from build123d import *

# Parameters (mm, degrees)
SCHIZZO1_W                   = 35
SCHIZZO1_H                   = 25
ESTRUSIONE_ESTRUSIONE1_DEPTH = 50
SCHIZZO2_R                   = 10.25
TAGLIO_ESTRUSIONE1_DEPTH     = 100
SCHIZZO3_R                   = 8.55
TAGLIO_ESTRUSIONE3_DEPTH     = 63.299678972
SMUSSO1_SIZE                 = 0.5


with BuildPart() as part:
    # Schizzo1 → Estrusione-Estrusione1 (new, symmetric)
    with BuildSketch(Plane.XY):
        Rectangle(SCHIZZO1_W, SCHIZZO1_H)
    extrude(amount=ESTRUSIONE_ESTRUSIONE1_DEPTH, both=True)

    # Schizzo2 → Taglio-Estrusione1 (cut)
    with BuildSketch(Plane(origin=(0, 12.5, 0), x_dir=(1, 0, 0), z_dir=(0, 1, 0))):
        with Locations(Location((0, 0, 0), (0, 0, 270))):
            Circle(SCHIZZO2_R)
    extrude(amount=-TAGLIO_ESTRUSIONE1_DEPTH, mode=Mode.SUBTRACT)

    # Schizzo3 → Taglio-Estrusione3 (cut, through all)
    with BuildSketch(Plane(origin=(17.5, 0, 0), x_dir=(0, 0, -1), z_dir=(1, 0, 0))):
        with Locations(Location((37.5, 0, 0), (0, 0, 90))):
            Circle(SCHIZZO3_R)
        with Locations(Location((-37.5, 0, 0), (0, 0, 90))):
            Circle(SCHIZZO3_R)
    extrude(amount=-TAGLIO_ESTRUSIONE3_DEPTH, mode=Mode.SUBTRACT)

    # Smusso1
    smusso1_edges = [part.edges().sort_by_distance(p)[0] for p in [
        (0, -12.5, -10.25),
        (0, 12.5, -10.25),
        (-17.5, -8.55, -37.5),
        (17.5, -8.55, -37.5),
        (-17.5, -8.55, 37.5),
        (17.5, -8.55, 37.5),
    ]]
    chamfer(smusso1_edges, length=SMUSSO1_SIZE)


solid = part.part
Read the model definition and answer for the solid it produces. Units are mm, in the model's axes. Round coordinates to 2 decimals unless told otherwise and drop trailing zeros. Loops run counter-clockwise (first coordinate to the right, second up) from the corner with the lowest first, then second, coordinate; pieces in that order, holes last.
Q1. Section D-D on x = -6 is taken. Give the number of separate pieces and of enclosed holes in the cut face, and give its area (3 significant figures).
Q2. Section A-A on y = 0 is taken. Write down the section's boundary in (x, z).
Q3. Consider probe 1 along X at (y, z) = (7, 0); probe 2 along Z at (x, y) = (5.5, -4); probe 3 along Z at (x, y) = (14, -7.75). Determine where each line is inside the solid, lowest interval first.
Q4. This flat-tipped pin is pushed along its axis until it touches: pin 1 (12.5 mm diameter, centred on x = 0, z = 0, fed in from -Y). Where does it stop, or does it pass through?
Q5. Section C-C on x = 15 is taken. Write down the section's boundary in (y, z).
Q6. Section B-B on z = 0 is taken. Write down the section's boundary in (x, y), and give its area (3 significant figures).
Q7. Determine the mould class of faces 1 (the face through (0, -12.5, 12)), 2 (the face through (-10.006, 0.168, -2.222)), 3 (the face through (0.238, -1.853, 29.153)), 4 (the face through (0.238, -1.853, -45.847)) for opening direction Y: released by +Y, released by -Y, zero draft, split by the parting line, or undercut.
Output:
1. separate pieces: 2
1. enclosed holes: 2
1. area: 1,620 mm2
2. outline: (-17.5, -50) - (17.5, -50) - (17.5, -46.55) - (17, -46.05) - (-17, -46.05) - (-17.5, -46.55) - close; (-17.5, -28.45) - (-17, -28.95) - (17, -28.95) - (17.5, -28.45) - (17.5, 28.45) - (17, 28.95) - (-17, 28.95) - (-17.5, 28.45) - close; (-17.5, 46.55) - (-17, 46.05) - (17, 46.05) - (17.5, 46.55) - (17.5, 50) - (-17.5, 50) - close; hole circle Ø20.5 at (0, 0)
3. probe 1: x = -17.5 to -10.25, 10.25 to 17.5
3. probe 2: z = -50 to -45.06, -29.94 to -8.65, 8.65 to 29.94, 45.06 to 50
3. probe 3: z = -50 to -41.11, -33.89 to 33.89, 41.11 to 50
4. pin 1: passes through
5. outline: (-12.5, -50) - (12.5, -50) - (12.5, 50) - (-12.5, 50) - close; hole circle Ø17.1 at (0, -37.5); hole circle Ø17.1 at (0, 37.5)
6. outline: (-17.5, -12.5) - (-10.75, -12.5) - (-10.25, -12) - (-10.25, 12) - (-10.75, 12.5) - (-17.5, 12.5) - close; (10.25, -12) - (10.75, -12.5) - (17.5, -12.5) - (17.5, 12.5) - (10.75, 12.5) - (10.25, 12) - close
6. area: 362 mm2
7. face 1: released by -Y
7. face 2: zero draft
7. face 3: undercut
7. face 4: undercut
